from build123d import *

# Parameters (mm, degrees)
PCB_START   = 32
SKETCH1_R   = 22.5
SKETCH1_R_2 = 15.85
PCB_DEPTH   = 1.6
LEDS_START  = 33.6
SKETCH2_W   = 5
SKETCH2_H   = 5
LEDS_DEPTH  = 1.6


with BuildPart() as part:
    # Sketch1 → PCB (new body)
    with BuildSketch(Plane(origin=(0, 0, 0), x_dir=(1, 0, 0), z_dir=(0, 1, 0)).offset(PCB_START)):
        with Locations(Location((0, 0, 0), (0, 0, 270))):
            Circle(SKETCH1_R)
        with Locations(Location((0, 0, 0), (0, 0, 270))):
            Circle(SKETCH1_R_2, mode=Mode.SUBTRACT)
    extrude(amount=PCB_DEPTH)

    # Sketch2 → LEDs (add)
    with BuildSketch(Plane(origin=(0, 0, 0), x_dir=(1, 0, 0), z_dir=(0, 1, 0)).offset(LEDS_START)):
        with Locations((19.175, 0)):
            Rectangle(SKETCH2_W, SKETCH2_H)
        Polygon((15.690973608, -6.172436491), (20.021100627, -8.672436491), (17.521100627, -13.002563509), (13.190973608, -10.502563509), align=None)
        Polygon((10.502563509, -13.190973608), (13.002563509, -17.521100627), (8.672436491, -20.021100627), (6.172436491, -15.690973608), align=None)
        with Locations((0, -19.175)):
            Rectangle(SKETCH2_W, SKETCH2_H)
        Polygon((-6.172436491, -15.690973608), (-8.672436491, -20.021100627), (-13.002563509, -17.521100627), (-10.502563509, -13.190973608), align=None)
        Polygon((-13.190973608, -10.502563509), (-17.521100627, -13.002563509), (-20.021100627, -8.672436491), (-15.690973608, -6.172436491), align=None)
        with Locations((-19.175, 0)):
            Rectangle(SKETCH2_W, SKETCH2_H)
        Polygon((-15.690973608, 6.172436491), (-20.021100627, 8.672436491), (-17.521100627, 13.002563509), (-13.190973608, 10.502563509), align=None)
        Polygon((-10.502563509, 13.190973608), (-13.002563509, 17.521100627), (-8.672436491, 20.021100627), (-6.172436491, 15.690973608), align=None)
        with Locations((0, 19.175)):
            Rectangle(SKETCH2_W, SKETCH2_H)
        Polygon((6.172436491, 15.690973608), (8.672436491, 20.021100627), (13.002563509, 17.521100627), (10.502563509, 13.190973608), align=None)
        Polygon((13.190973608, 10.502563509), (17.521100627, 13.002563509), (20.021100627, 8.672436491), (15.690973608, 6.172436491), align=None)
    extrude(amount=LEDS_DEPTH)


solid = part.part
Build history of the part. All positions in model axes, mm. A direction names the side the tool comes from. Give positions to 0.01 mm unless a question says otherwise; leave off trailing zeros. Order: outer loops, then holes, each group sorted by start corner. A loop starts at its lowest first (then second) coordinate and runs counter-clockwise, first axis right, second up. Notation, with made-up numbers: M 5.25,22.5 L 18.25,22.5 A20 ccw 18.25,30.5 Z; hole C 49.5,36 d9. An arc over 180 degrees is marked long. Use one line per item in the form item = value.
1) Saw through at A-A (x = 1). Give the cut face in (y, z) (3 decimals), plus the area to 3 significant figures.
Calculated:
outline = M 32,-22.478 L 33.6,-22.478 L 33.6,-21.675 L 35.2,-21.675 L 35.2,-16.675 L 33.6,-16.675 L 33.6,-15.818 L 32,-15.818 Z; M 32,15.818 L 33.6,15.818 L 33.6,16.675 L 35.2,16.675 L 35.2,21.675 L 33.6,21.675 L 33.6,22.478 L 32,22.478 Z
area = 37.3 mm2
2) Probe probe 1 along X at (y, z) = (32.5, 0); probe 2 along Z at (x, y) = (-18.5, 33.9); probe 3 along Z at (x, y) = (17, 34.8). List the from-to ranges inside material, lowest first.
Calculated:
probe_1 = -22.5 to -15.85, 15.85 to 22.5
probe_2 = -11.31 to -7.79, -2.5 to 2.5, 7.79 to 11.31
probe_3 = -12.7 to -6.93, -2.5 to 2.5, 6.93 to 12.7
3) Saw through at D-D (x = -4.5). Give the cut face in (y, z), plus the area to 3 significant figures.
Calculated:
outline = M 32,-22.05 L 33.6,-22.05 L 33.6,-15.2 L 32,-15.2 Z; M 32,15.2 L 33.6,15.2 L 33.6,22.05 L 32,22.05 Z
area = 21.9 mm2
4) Saw through at B-B (z = 0). Give the cut face in (x, y) (3 decimals).
Calculated:
outline = M -22.5,32 L -15.85,32 L -15.85,33.6 L -16.675,33.6 L -16.675,35.2 L -21.675,35.2 L -21.675,33.6 L -22.5,33.6 Z; M 15.85,32 L 22.5,32 L 22.5,33.6 L 21.675,33.6 L 21.675,35.2 L 16.675,35.2 L 16.675,33.6 L 15.85,33.6 Z
5) Tool access for faces 4 (the face through (14.42, 34.39, 8.37)), 5 (the face through (-19, 34, -2.5)), 6 (the face through (7.405, 34.389, -17.826)): list every direction of +Z, -Z, +X, -X, +Y, -Y with a clear straight run to the whole face (end or side of a thin tool).
Calculated:
face_4 = +Y
face_5 = +X, -X, +Y
face_6 = -Z, +Y
6) Saw through at C-C (y = 32.9). Give the cut face in (x, z).
Calculated:
outline = C 0,0 d45; hole C 0,0 d31.7
7) Two-plate mould, pull along X, no slides. Class faces 1 (the face through (-14.458, 34.389, 8.307)), 2 (the face through (10, 35.2, 17)), 3 (the face through (21.675, 34, 0)): released by +X, released by -X, zero draft, split by the parting line, or undercut.
Calculated:
face_1 = undercut
face_2 = zero draft
face_3 = released by +X
8) Drop flat-ended pins along their axis: pin 1 (1.5 mm diameter, centred on x = 16.5, z = -15, fed in from +Y); pin 2 (0.5 mm diameter, centred on y = 34.5, z = -0.5, fed in from +X) (3 decimals); pin 3 (1.3 mm diameter, centred on y = 34.5, z = 18, fed in from -X). Give the stop position or say it passes through.
Calculated:
pin_1 = 33.6
pin_2 = 21.675
pin_3 = -13
